Read the model definition and answer for the solid it produces. Units are mm, in the model's axes. Face numbers are marked on the shaded views. A direction names the side the tool comes from. Coordinates: 2 decimals unless noted, no trailing zeros. Order: outer loops, then holes, each group sorted by start corner. A loop starts at its lowest first (then second) coordinate and runs counter-clockwise, first axis right, second up. Notation, with made-up numbers: (14, -37) - (68, -37) arc R20 cw to (68, -6) - close; hole circle Ø9 at (4, 38). An arc over 180 degrees is marked (long way). Write item = value, one per line.
from build123d import *

# Parameters (mm, degrees)
SKETCH1_W               = 28
SKETCH1_H               = 33
FLANGE_DEPTH            = 5
NECK_START              = -14
SKETCH2_W               = 22
SKETCH2_H               = 27
NECK_DEPTH              = 14
PRONGS_START            = -25
SKETCH3_W               = 22
SKETCH3_H               = 27
PRONGS_DEPTH            = 11
SENSING_SLOT_DEPTH      = 34.064331235
SENSING_SLOT_DEPTH_BACK = 34.064331235
SKETCH4_W               = 10
SKETCH4_H               = 12
CABLE_STUB_START        = 5
SKETCH5_R               = 2
CABLE_STUB_DEPTH        = 15


with BuildPart() as part:
    # Sketch1 → Flange (new body)
    with BuildSketch(Plane(origin=(0, 0, 0), x_dir=(1, 0, 0), z_dir=(0, 1, 0))):
        Rectangle(SKETCH1_W, SKETCH1_H)
    extrude(amount=FLANGE_DEPTH)

    # Sketch2 → Neck (add)
    with BuildSketch(Plane(origin=(0, 0, 0), x_dir=(1, 0, 0), z_dir=(0, 1, 0)).offset(NECK_START)):
        Rectangle(SKETCH2_W, SKETCH2_H)
    extrude(amount=NECK_DEPTH)

    # Sketch3 → Prongs (add)
    with BuildSketch(Plane(origin=(0, 0, 0), x_dir=(1, 0, 0), z_dir=(0, 1, 0)).offset(PRONGS_START)):
        Rectangle(SKETCH3_W, SKETCH3_H)
    extrude(amount=PRONGS_DEPTH)

    # Sketch4 → Sensing_Slot (cut, two sides: drawn at the far end of the back side and taken through both)
    with BuildSketch(Plane.XY.offset(-SENSING_SLOT_DEPTH_BACK)):
        with Locations((0, -20)):
            Rectangle(SKETCH4_W, SKETCH4_H)
    extrude(amount=SENSING_SLOT_DEPTH + SENSING_SLOT_DEPTH_BACK, mode=Mode.SUBTRACT)

    # Sketch5 → Cable_Stub (add)
    with BuildSketch(Plane(origin=(0, 0, 0), x_dir=(1, 0, 0), z_dir=(0, 1, 0)).offset(CABLE_STUB_START)):
        with Locations(Location((0, 0, 0), (0, 0, 270))):
            Circle(SKETCH5_R)
    extrude(amount=CABLE_STUB_DEPTH)


solid = part.part
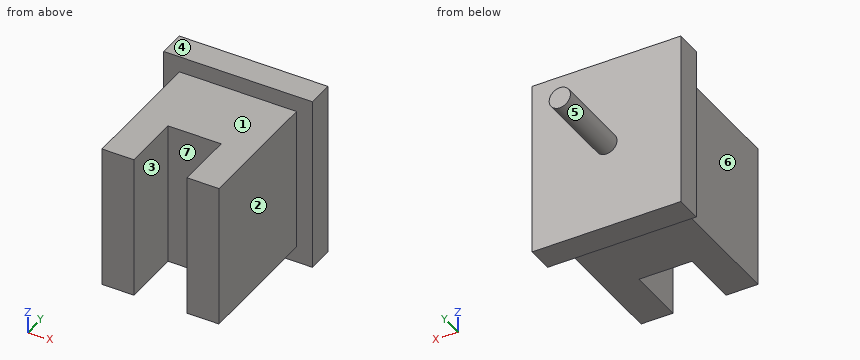
1) The part is cut by section B-B (x = -4.25). Determine the outline of the cut face in (y, z), and give its area (3 significant figures).
Returned:
outline = (-14, -13.5) - (0, -13.5) - (0, -16.5) - (5, -16.5) - (5, 16.5) - (0, 16.5) - (0, 13.5) - (-14, 13.5) - close
area = 543 mm^2
2) Flat-ended cylindrical pins translate along their axes: pin 1 Ø3.5 at (y, z) = (-22, -4) entering from -X; pin 2 Ø1 at (x, z) = (1.5, -4.5) entering from -Y; pin 3 Ø7.5 at (y, z) = (-10.5, 1) entering from +X. Find the tip coordinate at first contact, or state that the pin passes through.
Returned:
pin_1 = -11
pin_2 = -14
pin_3 = 11
3) The part is cut by section A-A (y = -16). Determine the outline of the cut face in (x, z), and give its area (3 significant figures).
Returned:
outline = (-11, -13.5) - (-5, -13.5) - (-5, 13.5) - (-11, 13.5) - close; (5, -13.5) - (11, -13.5) - (11, 13.5) - (5, 13.5) - close
area = 324 mm^2
4) Determine the mould class of the marked faces 4, 5, 6 and 7 for opening direction X: pulls with the +X half, pulls with the -X half, needs draft (parallel to the pull), parting line crosses it, or undercut.
Returned:
face_4 = needs draft
face_5 = parting line crosses it
face_6 = pulls with the -X half
face_7 = undercut
5) The part is cut by section D-D (z = 6). Determine the outline of the cut face in (x, y).
Returned:
outline = (-14, 0) - (-11, 0) - (-11, -25) - (-5, -25) - (-5, -14) - (5, -14) - (5, -25) - (11, -25) - (11, 0) - (14, 0) - (14, 5) - (-14, 5) - close
6) Straight lines are drawn through the part: line 1 along X through (y, z) = (-15, -10); line 2 along Z through (x, y) = (10.75, -9); line 3 along X through (y, z) = (-7, -13). For each, find the intervals that lie inside material, in ascending order. Write a range as from..to.
Returned:
line_1 = -11..-5, 5..11
line_2 = -13.5..13.5
line_3 = -11..11
7) The part is cut by section C-C (z = 0). Determine the outline of the cut face in (x, y), and give its area (3 significant figures).
Returned:
outline = (-14, 0) - (-11, 0) - (-11, -25) - (-5, -25) - (-5, -14) - (5, -14) - (5, -25) - (11, -25) - (11, 0) - (14, 0) - (14, 5) - (2, 5) - (2, 20) - (-2, 20) - (-2, 5) - (-14, 5) - close
area = 640 mm^2
8) For the marked faces 1, 2 and 3, determine the directions among +Z, -Z, +X, -X, +Y, -Y from which every point of the face is accessible in a straight line to the end or side of a thin tool.
Returned:
face_1 = +Z, +X, -X, -Y
face_2 = +Z, -Z, +X, -Y
face_3 = +Z, -Z, -Y
